from build123d import *

# Parameters (mm, degrees)
EXTRUDE_1_DEPTH              = 0.5
SKETCH_2_R                   = 2.5
EXTRUDE_2_DEPTH              = 21.5
HOLE_WIZARD_M3_1_D           = 2.5
HOLE_WIZARD_M3_1_DEPTH       = 7.5
HOLE_WIZARD_M3_1_CSINK_D     = 3
HOLE_WIZARD_M3_1_CSINK_ANGLE = 90
HOLE_WIZARD_M3_1_TIP         = 0.751075774


with BuildPart() as part:
    # 草图1 → 凸台-拉伸1 (new body)
    with BuildSketch(Plane(origin=(0, 0, 0), x_dir=(1, 0, 0), z_dir=(0, 1, 0))):
        Polygon((0, -3.175426481), (2.75, -1.58771324), (2.75, 1.58771324), (0, 3.175426481), (-2.75, 1.58771324), (-2.75, -1.58771324), align=None)
    extrude(amount=EXTRUDE_1_DEPTH)

    # 草图2 → 凸台-拉伸2 (add)
    with BuildSketch(Plane(origin=(0, 0.5, 0), x_dir=(1, 0, 0), z_dir=(0, 1, 0))):
        Circle(SKETCH_2_R)
    extrude(amount=EXTRUDE_2_DEPTH)

    # M3 螺纹孔1
    with Locations(Plane(origin=(0, 22, 0), x_dir=(1, 0, 0), z_dir=(0, 1, 0))):
        with Locations((0, 0)):
            CounterSinkHole(HOLE_WIZARD_M3_1_D / 2, HOLE_WIZARD_M3_1_CSINK_D / 2, depth=HOLE_WIZARD_M3_1_DEPTH, counter_sink_angle=HOLE_WIZARD_M3_1_CSINK_ANGLE)
            with Locations((0, 0, -(HOLE_WIZARD_M3_1_DEPTH + HOLE_WIZARD_M3_1_TIP / 2))):  # 118° drill point
                Cone(0, HOLE_WIZARD_M3_1_D / 2, HOLE_WIZARD_M3_1_TIP, mode=Mode.SUBTRACT)


solid = part.part
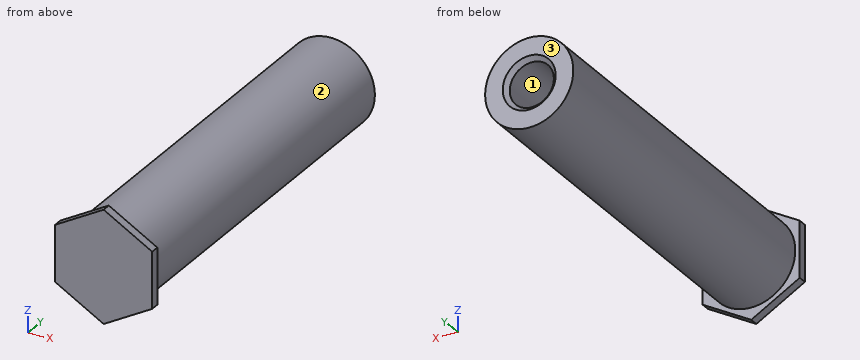
Check sheet for the modelled part. Datum: model origin and axes. Units: mm. Face numbers are marked on the shaded views. Coordinates: 2 decimals unless noted, no trailing zeros. Loops run counter-clockwise (first coordinate to the right, second up) from the corner with the lowest first, then second, coordinate; pieces in that order, holes last. Notation, with made-up numbers: (-7, -31) -> (-2, -31) arc R5 ccw to (-2, -24) -> close; hole circle Ø3 at (77, 42.5). An arc over 180 degrees is marked (long way). Write item = value, one per line. Start each with the question number.
1. Section check A-A on y = 20.75. Record the cut outline in (x, z), then the cut area to 3 significant figures.
2. Draft check along Z on the marked faces 1, 2 and 3. Enter one of: released by +Z, released by -Z, zero draft, split by the parting line, or undercut.
3. Depth check by flat-ended pin: P1, Ø3, axis at x = 0, z = 0, coming from the -Y side; P2, Ø2, axis at x = 0, y = 8.5, coming from the -Z side. Enter the tip coordinate at first touch or a pass-through.
4. Material ranges on line 1 (Z direction, x = 0, y = 19); line 2 (Y direction, x = -2.4, z = -1); line 3 (Z direction, x = -0.55, y = 18.25), recorded low to high.
5. Section check B-B on y = 10.25. Record the cut outline in (x, z), then the cut area to 3 significant figures.
Responses:
q1.outline = circle Ø5 at (0, 0); hole circle Ø2.5 at (0, 0)
q1.area = 14.7 mm2
q2.face_1 = undercut
q2.face_2 = split by the parting line
q2.face_3 = zero draft
q3.P1 = 0
q3.P2 = -2.5
q4.line_1 = -2.5 to -1.25, 1.25 to 2.5
q4.line_2 = 0 to 0.5
q4.line_3 = -2.44 to -1.12, 1.12 to 2.44
q5.outline = circle Ø5 at (0, 0)
q5.area = 19.6 mm2
